from build123d import *

# Parameters (mm, degrees)
SKETCH1_W           = 1.6
SKETCH1_H           = 8.4
SKETCH1_H_2         = 1.6
SKETCH1_H_3         = 10
BOSS_EXTRUDE1_DEPTH = 6
FILLET1_R           = 1
FILLET2_R           = 2


with BuildPart() as part:
    # Sketch1 → Boss-Extrude1 (new body)
    with BuildSketch(Plane(origin=(0, 0, 0), x_dir=(1, 0, 0), z_dir=(0, 1, 0))):
        with Locations((-246.2, 65.3)):
            Rectangle(SKETCH1_W, SKETCH1_H)
        with Locations((-246.2, 60.3)):
            Rectangle(SKETCH1_W, SKETCH1_H_2)
        with BuildLine():
            Line((-245.4, 59.5), (-17, 59.5))
            ThreePointArc((-17, 59.5), (-12.917127972, 57.896607329), (-11.016404973, 53.943385336))
            Line((-11.016404973, 53.943385336), (-6.980860865, -0.517282892))
            ThreePointArc((-6.980860865, -0.517282892), (0.324323403, -6.992482701), (6.998771924, 0.131116578))
            Line((6.998771924, 0.131116578), (6.001052637, 53.387614362))
            ThreePointArc((6.001052637, 53.387614362), (7.717809332, 57.702718535), (12, 59.5))
            Line((12, 59.5), (241.4, 59.5))
            Line((241.4, 59.5), (241.4, 61.1))
            Line((241.4, 61.1), (12, 61.1))
            ThreePointArc((12, 61.1), (6.575891821, 58.823443478), (4.40133334, 53.357644858))
            Line((4.40133334, 53.357644858), (5.399052627, 0.101147074))
            ThreePointArc((5.399052627, 0.101147074), (0.250192339, -5.394200941), (-5.385235524, -0.399046802))
            Line((-5.385235524, -0.399046802), (-9.420779633, 54.061621425))
            ThreePointArc((-9.420779633, 54.061621425), (-11.828362098, 59.06903595), (-17, 61.1))
            Line((-17, 61.1), (-245.4, 61.1))
            Line((-245.4, 61.1), (-245.4, 59.5))
        make_face()
        with Locations((242.2, 60.3)):
            Rectangle(SKETCH1_W, SKETCH1_H_2)
        with Locations((242.2, 66.1)):
            Rectangle(SKETCH1_W, SKETCH1_H_3)
    extrude(amount=BOSS_EXTRUDE1_DEPTH)

    # Fillet1
    fillet1_edges = [part.edges().sort_by_distance(p)[0] for p in [
        (-245.4, 3, -61.1),
        (241.4, 3, -61.1),
    ]]
    fillet(fillet1_edges, radius=FILLET1_R)

    # Fillet2
    fillet2_edges = [part.edges().sort_by_distance(p)[0] for p in [
        (243, 3, -59.5),
        (-247, 3, -59.5),
    ]]
    fillet(fillet2_edges, radius=FILLET2_R)


solid = part.part
Design review of the part built by this model. Coordinates are the model's own, in mm. Give positions to 0.01 mm unless a question says otherwise; leave off trailing zeros. Loops run counter-clockwise (first coordinate to the right, second up) from the corner with the lowest first, then second, coordinate; pieces in that order, holes last. Notation, with made-up numbers: M -20,72 L 3,72 A18 ccw 3,76 Z; hole C 75,13.25 d9. An arc over 180 degrees is marked long. One line per question, with ' | ' between items. Start each with the question number.
1. Insertion check: P1, Ø3, axis at x = -124, y = 2.5, coming from the -Z side; P2, Ø1.8, axis at x = 120.5, y = 3.5, coming from the +Z side; P3, Ø1.8, axis at x = -246.5, y = 2, coming from the -Z side. Each pin has a flat end and moves straight along its axis. Give the tip position at first contact, or say it passes through.
2. Add section A-A (y = 4.2). Write out the cut boundary in (x, z).
3. Add section B-B (z = -34). Write out the cut boundary in (x, y), plus the area to 3 significant figures.
4. Add section C-C (x = 0). Write out the cut boundary in (y, z).
5. To check wall thickness, follow L1, parallel to X at y = 1.2, z = -67; L2, parallel to X at y = 2.15, z = -54.5; L3, parallel to Z at x = -105, y = 0.95. State the ranges of each line that lie inside material, in increasing order.
Worked out:
1) P1: stops at z = -61.1 | P2: stops at z = -59.5 | P3: stops at z = -69.5
2) outline: M -247,-69.5 L -245.4,-69.5 L -245.4,-62.1 A1 cw -244.4,-61.1 L -17,-61.1 A7.6 ccw -9.42,-54.06 L -5.39,0.4 A5.4 cw 5.4,-0.1 L 4.4,-53.36 A7.6 ccw 12,-61.1 L 240.4,-61.1 A1 cw 241.4,-62.1 L 241.4,-71.1 L 243,-71.1 L 243,-61.5 A2 ccw 241,-59.5 L 12,-59.5 A6 cw 6,-53.39 L 7,-0.13 A7 ccw -6.98,0.52 L -11.02,-53.94 A6 cw -17,-59.5 L -245,-59.5 A2 ccw -247,-61.5 Z
3) outline: M -9.54,0 L -7.93,0 L -7.93,6 L -9.54,6 Z; M 4.76,0 L 6.36,0 L 6.36,6 L 4.76,6 Z | area: 19.2 mm²
4) outline: M 0,5.4 L 6,5.4 L 6,7 L 0,7 Z
5) L1: x = -247 to -245.4, 241.4 to 243 | L2: x = -11.08 to -9.47, 4.47 to 6.08 | L3: z = -61.1 to -59.5
